Geometry: final body of the model. Coordinates: model frame, mm. A direction names the side the tool comes from. Coordinates: 2 decimals unless noted, no trailing zeros. Write each loop counter-clockwise with the first axis right and the second up, starting at its lowest first coordinate (ties: lowest second). Pieces come first, ordered by that corner, then holes. Notation, with made-up numbers: (61, -38) - (111, -38) arc R32 cw to (111, -4) - close; hole circle Ø5 at (-14, -15). An arc over 180 degrees is marked (long way). Answer as a JSON object with one key per item and string values. Group by question number.
Item 1: Set-up query: faces 1 (the flat face through (-34, 10.16, -90)), 2 (the flat face through (-24.6, 5, -34)). Return all of +Z, -Z, +X, -X, +Y, -Y with unobstructed straight access to the full face (end or side cutting, diameter ignored); none if empty.
Item 2: Line query: line 1 along X through (y, z) = (5.25, 11); line 2 along Z through (x, y) = (24, 6); line 3 along Z through (x, y) = (-6, 2). Output: solid intervals per line, ascending. Write a range as from..to.
Item 3: Section B-B on x = -37.3. Return loops of the section in (y, z), and give its area (3 significant figures).
Item 4: Mould query, pull axis X, two halves, no side actions, for faces 3 (the flat face through (-50, 5, -45)), 4 (the cylindrical face through (-38.516, 5.151, -48.131)), 5 (the flat face through (11, 5, -102.626)). Classes: pulls with the +X half, pulls with the -X half, needs draft (parallel to the pull), parting line crosses it, or undercut.
Item 5: Section A-A on y = 5.75. Return loops of the section in (x, z) (3 decimals), and give its area (4 significant figures).
Item 6: First-contact query: pin 1 Ø5 at (x, y) = (17.5, 4.5) entering from +Z; pin 2 Ø3 at (y, z) = (2.5, -62) entering from +X. Flat tips, straight axial feed; report the tip coordinate or a pass-through.
Item 7: Section C-C on z = -79. Return loops of the section in (x, y).
Item 8: Section D-D on x = 18. Return loops of the section in (y, z), and give its area (3 significant figures).
```python
from build123d import *

# Parameters (mm, degrees)
BOSS_EXTRUDE1_DEPTH = 10.16
SKETCH2_R           = 3.175
CUT_EXTRUDE1_DEPTH  = 10.16
FILLET1_R           = 2.54


with BuildPart() as part:
    # Sketch1 → Boss-Extrude1 (new body)
    with BuildSketch(Plane(origin=(0, 0, 0), x_dir=(1, 0, 0), z_dir=(0, 1, 0))):
        Polygon((-50, 128.026), (42.202, 166.126), (42.202, 128.026), (42.202, 102.626), (-24.6, 102.626), (-24.6, -34.28), (-50, -34.28), align=None)
    extrude(amount=BOSS_EXTRUDE1_DEPTH)

    # Sketch2 → Cut-Extrude1 (cut)
    with BuildSketch(Plane(origin=(0, 10.16, 0), x_dir=(1, 0, 0), z_dir=(0, 1, 0))):
        with Locations(Location((-37.3, 51.064, 0), (0, 0, 270))):
            Circle(SKETCH2_R)
    extrude(amount=-CUT_EXTRUDE1_DEPTH, mode=Mode.SUBTRACT)

    # Fillet1
    fillet1_edges = [part.edges().sort_by_distance(p)[0] for p in [
        (-50, 5.08, -128.026),
        (-24.6, 5.08, -102.626),
    ]]
    fillet(fillet1_edges, radius=FILLET1_R)


solid = part.part
```
Checks:
{
 "1": {"face 1": "+Z, -Z, +X, -X, +Y", "face 2": "+Z, +X, +Y, -Y"},
 "2": {"line 1": "-50..-24.6", "line 2": "-158.6..-102.63", "line 3": "-146.21..-102.63"},
 "3": {"outline": "(0, -133.27) - (10.16, -133.27) - (10.16, -54.24) - (0, -54.24) - close; (0, -47.89) - (10.16, -47.89) - (10.16, 34.28) - (0, 34.28) - close", "area": "1,640 mm^2"},
 "4": {"face 3": "pulls with the -X half", "face 4": "undercut", "face 5": "needs draft"},
 "5": {"outline": "(-50, -126.327) arc R2.54 ccw to (-48.43, -128.675) - (42.202, -166.126) - (42.202, -102.626) - (-22.06, -102.626) arc R2.54 cw to (-24.6, -100.086) - (-24.6, 34.28) - (-50, 34.28) - close; hole circle Ø6.35 at (-37.3, -51.064)", "area": "7,545 mm^2"},
 "6": {"pin 1": "z = -102.63", "pin 2": "x = -24.6"},
 "7": {"outline": "(-50, 0) - (-24.6, 0) - (-24.6, 10.16) - (-50, 10.16) - close"},
 "8": {"outline": "(0, -156.13) - (10.16, -156.13) - (10.16, -102.63) - (0, -102.63) - close", "area": "544 mm^2"}
}
